Geometry check sheet. Reference: the model listing, model coordinates, mm. Face numbers are marked on the shaded views. Give positions to 0.01 mm unless a question says otherwise; leave off trailing zeros. Loops run counter-clockwise (first coordinate to the right, second up) from the corner with the lowest first, then second, coordinate; pieces in that order, holes last.
1. Material ranges on L1, parallel to Y at x = -142.5, z = 8; L2, parallel to Y at x = -97, z = 10.5; L3, parallel to Z at x = -93.5, y = -27, recorded low to high.
2. Release check for a two-part mould opening along Z. For the marked faces 1, 2 and 3 record: +Z half, -Z half, draft (parallel to the pull), parting line (faces both ways), or undercut.
3. Go/stop test with flat-tipped pins: pin 1 Ø4 at (x, z) = (-90, 9) entering from +Y; pin 2 Ø20 at (x, y) = (-136, 8) entering from +Z; pin 3 Ø3 at (y, z) = (-1, 7) entering from +X; pin 4 Ø1 at (y, z) = (-26.5, 6.5) entering from +X. Record where each tip stops, or that it passes through.
4. Cross-section at C-C, the plane x = -142.5. Record the cut outline in (y, z).
5. Cross-section at D-D, the plane y = -27.5. Record the cut outline in (x, z), plus the area to 3 significant figures.
6. Cross-section at A-A, the plane z = 6.75. Record the cut outline in (x, y).
7. Cross-section at B-B, the plane y = 6.5. Record the cut outline in (x, z), plus the area to 3 significant figures.
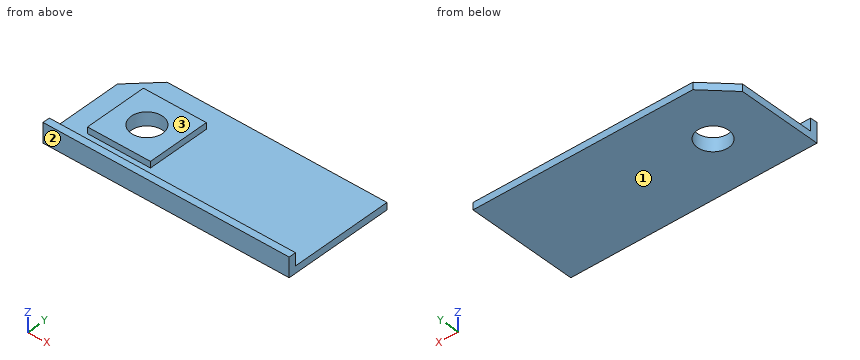
from build123d import *

# Parameters (mm, degrees)
SKETCH2_R           = 10
BOSS_EXTRUDE2_DEPTH = 4.5
SKETCH2_5_W         = 90
SKETCH2_5_H         = 65.5
BOSS_EXTRUDE4_DEPTH = 4.5
BOSS_EXTRUDE5_DEPTH = 12.5
SKETCH4_W           = 40
SKETCH4_H           = 40
SKETCH4_R           = 10
BOSS_EXTRUDE6_DEPTH = 4


with BuildPart() as part:
    # Sketch2 → Boss-Extrude2 (new body)
    with BuildSketch(Plane(origin=(0, 0, 0), x_dir=(-1, 0, 0), z_dir=(0, 0, 1))):
        Polygon((96.758646955, 28.875433948), (96.758646955, -36.624566052), (146.427679381, -36.624566052), (163.18445937, -19.867786064), (163.18445937, 28.875433948), align=None)
        with Locations(Location((128.427679381, -1.867786064, 0), (0, 0, 180))):
            Circle(SKETCH2_R, mode=Mode.SUBTRACT)
    extrude(amount=BOSS_EXTRUDE2_DEPTH)

    # Sketch2_5 → Boss-Extrude4 (add)
    with BuildSketch(Plane(origin=(0, 0, 0), x_dir=(-1, 0, 0), z_dir=(0, 0, 1))):
        with Locations((51.758646955, -3.874566052)):
            Rectangle(SKETCH2_5_W, SKETCH2_5_H)
    extrude(amount=BOSS_EXTRUDE4_DEPTH)

    # Sketch2_7 → Boss-Extrude5 (add)
    with BuildSketch(Plane(origin=(0, 0, 0), x_dir=(-1, 0, 0), z_dir=(0, 0, 1))):
        Polygon((6.758646955, 33.375433948), (6.758646955, 28.875433948), (96.758646955, 28.875433948), (163.18445937, 28.875433948), (163.18445937, 33.375433948), align=None)
    extrude(amount=BOSS_EXTRUDE5_DEPTH)

    # Sketch4 → Boss-Extrude6 (add)
    with BuildSketch(Plane.XY.offset(4.5)):
        with Locations((-128.427679381, 1.867786064)):
            Rectangle(SKETCH4_W, SKETCH4_H)
        with Locations((-128.427679381, 1.867786064)):
            Circle(SKETCH4_R, mode=Mode.SUBTRACT)
    extrude(amount=BOSS_EXTRUDE6_DEPTH)


solid = part.part
Result:
1. L1: y = -33.38 to -28.88, -18.13 to 21.87
1. L2: y = -33.38 to -28.88
1. L3: z = 0 to 4.5
2. face 1: -Z half
2. face 2: draft
2. face 3: +Z half
3. pin 1: stops at y = -28.88
3. pin 2: stops at z = 8.5
3. pin 3: stops at x = -108.43
3. pin 4: passes through
4. outline: (-33.38, 0) - (36.62, 0) - (36.62, 4.5) - (21.87, 4.5) - (21.87, 8.5) - (-18.13, 8.5) - (-18.13, 4.5) - (-28.88, 4.5) - (-28.88, 12.5) - (-33.38, 12.5) - close
5. outline: (-163.18, 0) - (-6.76, 0) - (-6.76, 4.5) - (-163.18, 4.5) - close
5. area: 704 mm2
6. outline: (-163.18, -33.38) - (-6.76, -33.38) - (-6.76, -28.88) - (-163.18, -28.88) - close; (-148.43, -18.13) - (-108.43, -18.13) - (-108.43, 21.87) - (-148.43, 21.87) - close; hole circle Ø20 at (-128.43, 1.87)
7. outline: (-163.18, 0) - (-137.29, 0) - (-137.29, 8.5) - (-148.43, 8.5) - (-148.43, 4.5) - (-163.18, 4.5) - close; (-119.57, 0) - (-6.76, 0) - (-6.76, 4.5) - (-108.43, 4.5) - (-108.43, 8.5) - (-119.57, 8.5) - close
7. area: 713 mm2
